The model under review builds one solid part; all positions refer to its coordinate system, in mm. A direction names the side the tool comes from. Coordinates: 2 decimals unless noted, no trailing zeros. Write each loop counter-clockwise with the first axis right and the second up, starting at its lowest first coordinate (ties: lowest second). Pieces come first, ordered by that corner, then holes. Notation, with made-up numbers: (25, 69) - (52, 69) arc R31 cw to (52, 96) - close; hole circle Ø5 at (80, 1.5). An arc over 180 degrees is marked (long way). Put each result on its own line as item: value. Start each with the question number.
Item 1: Consider section A-A on z = -5.5. Give the boundary of the cut face in (x, y) (3 decimals), then the cut area to 3 significant figures.
Item 2: Mouldability with a two-part tool opening along Y and no side actions: class faces 3 (the face through (2, -20, -2.54)), 4 (the face through (3.175, -20, 10)), 5 (the face through (2, -6.985, 9)) as pulls with the +Y half, pulls with the -Y half, needs draft (parallel to the pull), parting line crosses it, or undercut.
Item 3: Consider section B-B on y = -12.7. Give the boundary of the cut face in (x, z) (3 decimals), then the cut area to 3 significant figures.
Item 4: To check wall thickness, follow L1, parallel to Y at x = 1.8, z = 12.7 (3 decimals); L2, parallel to Z at x = 3, y = -21 (3 decimals); L3, parallel to Z at x = 2.95, y = -21.75 (3 decimals). State the ranges of each line that lie inside material, in increasing order. Write a range as [from, to].
Item 5: Machinability: for faces 1 (the face through (2, -20, 34.925)), 2 (the face through (2, -23.495, -6)), which of the approach directions +Z, -Z, +X, -X, +Y, -Y give a long, thin tool a straight path to every point of the face, cutting with its end or side? Answer none if there is none.
Item 6: Consider section C-C on x = 2.4. State how many separate pieces and enclosed holes the cut face has, then the cut area to 3 significant figures.
```python
from build123d import *

# Parameters (mm, degrees)
SKETCH1_W           = 24.765
SKETCH1_H           = 50.8
SKETCH1_R           = 1.75
SKETCH1_W_2         = 6.35
SKETCH1_H_2         = 6.35
BOSS_EXTRUDE1_DEPTH = 3.175
FILLET1_R           = 0.79375


with BuildPart() as part:
    # Sketch1 → Boss-Extrude1 (new body)
    with BuildSketch(Plane.YZ):
        with Locations((-19.3675, 9.525)):
            Rectangle(SKETCH1_W, SKETCH1_H)
        with Locations(Location((-27.225, -9.525, 0), (0, 0, 270))):
            Circle(SKETCH1_R, mode=Mode.SUBTRACT)
        with Locations((-20.32, -5.715)):
            Rectangle(SKETCH1_W_2, SKETCH1_H_2, mode=Mode.SUBTRACT)
        with Locations(Location((-12.7, 12.7, 0), (0, 0, 270))):
            Circle(SKETCH1_R, mode=Mode.SUBTRACT)
        with Locations(Location((-22.225, 25.4, 0), (0, 0, 270))):
            Circle(SKETCH1_R, mode=Mode.SUBTRACT)
    extrude(amount=BOSS_EXTRUDE1_DEPTH)

    # Fillet1
    fillet1_edges = [part.edges().sort_by_distance(p)[0] for p in [
        (1.5875, -23.495, -2.54),
        (1.5875, -23.495, -8.89),
        (1.5875, -17.145, -8.89),
        (1.5875, -17.145, -2.54),
        (1.5875, -6.985, -15.875),
        (1.5875, -31.75, -15.875),
        (1.5875, -31.75, 34.925),
        (1.5875, -6.985, 34.925),
    ]]
    fillet(fillet1_edges, radius=FILLET1_R)


solid = part.part
```
Report:
1. outline: (0, -31.75) - (3.175, -31.75) - (3.175, -23.495) - (0, -23.495) - close; (0, -17.145) - (3.175, -17.145) - (3.175, -6.985) - (0, -6.985) - close
1. area: 58.5 mm²
2. face 3: undercut
2. face 4: needs draft
2. face 5: pulls with the +Y half
3. outline: (0, -15.875) - (3.175, -15.875) - (3.175, 10.95) - (0, 10.95) - close; (0, 14.45) - (3.175, 14.45) - (3.175, 34.925) - (0, 34.925) - close
3. area: 150 mm²
4. L1: [-31.75, -14.45], [-10.95, -6.985]
4. L2: [-15.875, -8.89], [-2.54, 24.15], [26.65, 34.925]
4. L3: [-15.875, -8.89], [-2.54, 23.716], [27.084, 34.925]
5. face 1: +Z, +X, -X, +Y, -Y
5. face 2: +X, -X
6. separate pieces: 1
6. enclosed holes: 4
6. area: 1,190 mm²
